Design review of the part built by this model. Coordinates are the model's own, in mm. Coordinates: 2 decimals unless noted, no trailing zeros. Loops run counter-clockwise (first coordinate to the right, second up) from the corner with the lowest first, then second, coordinate; pieces in that order, holes last. Notation, with made-up numbers: (21, 20) -> (50, 20) arc R32 ccw to (50, 58) -> close; hole circle Ø10 at (-4.75, 6.25). An arc over 180 degrees is marked (long way). Answer in a Markdown table with one row per item.
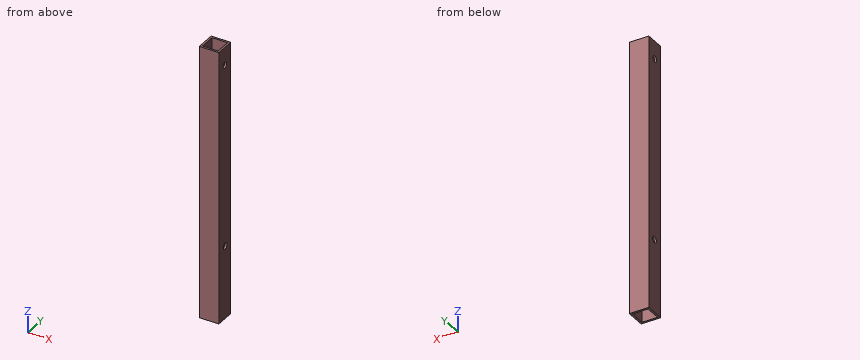
```python
from build123d import *

# Parameters (mm, degrees)
SKETCH_1_W          = 10
SKETCH_1_H          = 10
SKETCH_1_W_2        = 8
SKETCH_1_H_2        = 8
EXTRUDE_1_DEPTH     = 140
SKETCH_2_R          = 1.6
CUT_EXTRUDE_1_DEPTH = 141.445719052
SKETCH_3_R          = 1.6
CUT_EXTRUDE_2_DEPTH = 141.445719052


with BuildPart() as part:
    # ｽｹｯﾁ1 → ﾎﾞｽ - 押し出し1 (new body)
    with BuildSketch(Plane.XY):
        Rectangle(SKETCH_1_W, SKETCH_1_H)
        Rectangle(SKETCH_1_W_2, SKETCH_1_H_2, mode=Mode.SUBTRACT)
    extrude(amount=EXTRUDE_1_DEPTH)

    # ｽｹｯﾁ2 → ｶｯﾄ - 押し出し1 (cut, through all)
    with BuildSketch(Plane(origin=(5, 0, 0), x_dir=(0, 0, -1), z_dir=(1, 0, 0))):
        with Locations(Location((-130.81, 0, 0), (0, 0, 90))):
            Circle(SKETCH_2_R)
    extrude(amount=-CUT_EXTRUDE_1_DEPTH, mode=Mode.SUBTRACT)

    # ｽｹｯﾁ3 → ｶｯﾄ - 押し出し2 (cut, through all)
    with BuildSketch(Plane(origin=(5, 0, 0), x_dir=(0, 0, -1), z_dir=(1, 0, 0))):
        with Locations(Location((-37.465120214, 0.258526647, 0), (0, 0, 90))):
            Circle(SKETCH_3_R)
    extrude(amount=-CUT_EXTRUDE_2_DEPTH, mode=Mode.SUBTRACT)


solid = part.part
```
(1) Take a section at D-D on z = 43.5. Give the boundary of the cut face in (x, y).
Evaluation:
| item | result |
|---|---|
| outline | (-5, -5) -> (5, -5) -> (5, 5) -> (-5, 5) -> close; hole (-4, -4) -> (4, -4) -> (4, 4) -> (-4, 4) -> close |
(2) Take a section at B-B on z = 130.81. Give the boundary of the cut face in (x, y), and give its area (3 significant figures).
Evaluation:
| item | result |
|---|---|
| outline | (-5, -5) -> (5, -5) -> (5, -1.6) -> (4, -1.6) -> (4, -4) -> (-4, -4) -> (-4, -1.6) -> (-5, -1.6) -> close; (-5, 1.6) -> (-4, 1.6) -> (-4, 4) -> (4, 4) -> (4, 1.6) -> (5, 1.6) -> (5, 5) -> (-5, 5) -> close |
| area | 29.6 mm² |
(3) Take a section at A-A on x = -1.25. Give the boundary of the cut face in (y, z), and give its area (3 significant figures).
Evaluation:
| item | result |
|---|---|
| outline | (-5, 0) -> (-4, 0) -> (-4, 140) -> (-5, 140) -> close; (4, 0) -> (5, 0) -> (5, 140) -> (4, 140) -> close |
| area | 280 mm² |
(4) Take a section at C-C on y = 0. Give the boundary of the cut face in (x, z).
Evaluation:
| item | result |
|---|---|
| outline | (-5, 0) -> (-4, 0) -> (-4, 35.89) -> (-5, 35.89) -> close; (-5, 39.04) -> (-4, 39.04) -> (-4, 129.21) -> (-5, 129.21) -> close; (-5, 132.41) -> (-4, 132.41) -> (-4, 140) -> (-5, 140) -> close; (4, 0) -> (5, 0) -> (5, 35.89) -> (4, 35.89) -> close; (4, 39.04) -> (5, 39.04) -> (5, 129.21) -> (4, 129.21) -> close; (4, 132.41) -> (5, 132.41) -> (5, 140) -> (4, 140) -> close |
(5) To check wall thickness, follow probe 1 along Z at (x, y) = (-4.3, 0); probe 2 along Y at (x, z) = (0, 28.5). State the ranges of each line that lie inside material, in increasing order.
Evaluation:
| item | result |
|---|---|
| probe 1 | z = 0 to 35.89, 39.04 to 129.21, 132.41 to 140 |
| probe 2 | y = -5 to -4, 4 to 5 |
